```python
from build123d import *

# Parameters (mm, degrees)
EXTRUDE_1_DEPTH     = 5
EXTRUDE_5_DEPTH     = 30
EXTRUDE_6_DEPTH     = 30
CUT_EXTRUDE_1_DEPTH = 50
EXTRUDE_7_DEPTH     = 10
EXTRUDE_9_DEPTH     = 100
CUT_EXTRUDE_2_DEPTH = 653.725056973
SKETCH_15_W         = 153.587108834
SKETCH_15_H         = 200
EXTRUDE_11_DEPTH    = 5


with BuildPart() as part:
    # 草图1 → 凸台-拉伸1 (new body)
    with BuildSketch(Plane(origin=(0, 0, 0), x_dir=(1, 0, 0), z_dir=(0, 1, 0))):
        Polygon((-505, -50), (-505, 220), (-425, 300), (425, 300), (505, 220), (505, -10), (505, -220), (425, -300), (-425, -300), (-505, -220), align=None)
    extrude(amount=EXTRUDE_1_DEPTH)

    # 草图5 → 凸台-拉伸5 (add)
    with BuildSketch(Plane(origin=(0, 5, 0), x_dir=(1, 0, 0), z_dir=(0, 1, 0))):
        Polygon((90, 0), (90, -10), (110, -10), (110, 10), (90, 10), align=None)
    extrude(amount=EXTRUDE_5_DEPTH)

    # 草图6 → 凸台-拉伸6 (add)
    with BuildSketch(Plane(origin=(0, 35, 0), x_dir=(1, 0, 0), z_dir=(0, 1, 0))):
        Polygon((100, -25), (125, -25), (125, 25), (75, 25), (75, -25), align=None)
    extrude(amount=EXTRUDE_6_DEPTH)

    # 草图7 → 切除-拉伸1 (cut)
    with BuildSketch(Plane(origin=(125, 0, 0), x_dir=(0, 0, -1), z_dir=(1, 0, 0))):
        Polygon((0, 57.5), (-7.5, 57.5), (-7.5, 42.5), (7.5, 42.5), (7.5, 57.5), align=None)
    extrude(amount=-CUT_EXTRUDE_1_DEPTH, mode=Mode.SUBTRACT)

    # 草图8 → 凸台-拉伸7 (add)
    with BuildSketch(Plane(origin=(0, 5, 0), x_dir=(1, 0, 0), z_dir=(0, 1, 0))):
        with BuildLine():
            Line((505, 0), (505, 150))
            Line((505, 150), (424.355957742, 150))
            ThreePointArc((424.355957742, 150), (480, 0), (424.355957742, -150))
            Line((424.355957742, -150), (505, -150))
            Line((505, -150), (505, 0))
        make_face()
    extrude(amount=EXTRUDE_7_DEPTH)

    # 草图12 → 凸台-拉伸9 (add)
    with BuildSketch(Plane(origin=(0, 5, 0), x_dir=(1, 0, 0), z_dir=(0, 1, 0))):
        Polygon((30, -90), (100, -90), (180, -90), (180, -100), (100, -100), (30, -100), align=None)
        Polygon((100, 100), (30, 100), (30, 90), (100, 90), (180, 90), (180, 100), align=None)
    extrude(amount=EXTRUDE_9_DEPTH)

    # 草图13 → 切除-拉伸2 (cut, through all)
    with BuildSketch(Plane.XY.offset(100)):
        Polygon((180, 105), (180, 72), (30, 105), align=None)
    extrude(amount=-CUT_EXTRUDE_2_DEPTH, mode=Mode.SUBTRACT)

    # 草图15 → 凸台-拉伸11 (add)
    with BuildSketch(Plane(origin=(23.418542541, 106.447920641, 0), x_dir=(0.9766444667050901, -0.21486178267511977, 0), z_dir=(0.21486178267511977, 0.9766444667050901, 0))):
        with Locations((83.532401237, 0)):
            Rectangle(SKETCH_15_W, SKETCH_15_H)
    extrude(amount=EXTRUDE_11_DEPTH)


solid = part.part
```
The model under review builds one solid part; all positions refer to its coordinate system, in mm. A direction names the side the tool comes from. Round coordinates to 2 decimals unless told otherwise and drop trailing zeros. Loops run counter-clockwise (first coordinate to the right, second up) from the corner with the lowest first, then second, coordinate; pieces in that order, holes last. Notation, with made-up numbers: M 89.5,-3 L 99.5,-3 A34 ccw 99.5,32 Z; hole C 31,20.25 d4. An arc over 180 degrees is marked long. Put each result on its own line as item: value.
Q1. Machinability: for faces 1 (the flat face through (105.024, 93.614, -1.4)), 2 (the flat face through (100, 20, 10)), 3 (the flat face through (100, 65, 0)), 4 (the flat face through (89, 35, 0)), 5 (the flat face through (-464, 2, 261)), which of the approach directions +Z, -Z, +X, -X, +Y, -Y give a long, thin tool a straight path to every point of the face, cutting with its end or side? Answer none if there is none.
Result set:
face 1: +Z, -Z, +X, +Y
face 2: -X
face 3: +X, -X
face 4: none
face 5: +Z, -X, +Y, -Y
Q2. Consider section B-B, the plane z = 79. Give the boundary of the cut face in (x, y), then the cut area to 3 significant figures.
Result set:
outline: M -505,0 L 505,0 L 505,15 L 466.01,15 L 466.01,5 L -505,5 Z; M 30,105 L 180,72 L 181.07,76.88 L 31.07,109.88 Z
area: 6,210 mm²
Q3. Mouldability with a two-part tool opening along X and no side actions: class faces 6 (the flat face through (100, 20, -10)), 7 (the flat face through (110, 20, 0)), 8 (the flat face through (466, 2, 259)) as released by +X, released by -X, zero draft, split by the parting line, or undercut.
Result set:
face 6: zero draft
face 7: undercut
face 8: released by +X
Q4. Consider section D-D, the plane z = 204. Give the boundary of the cut face in (x, y), then the cut area to 3 significant figures.
Result set:
outline: M -505,0 L 505,0 L 505,5 L -505,5 Z
area: 5,050 mm²
Q5. Consider section C-C, the plane x = -274.5. Give the boundary of the cut face in (y, z), then the cut area to 3 significant figures.
Result set:
outline: M 0,-300 L 5,-300 L 5,300 L 0,300 Z
area: 3,000 mm²
Q6. For pin 1 (6 mm diameter, centred on y = 20.5, z = 2.5, fed in from +X); pin 2 (8 mm diameter, centred on y = 67, z = -96, fed in from -X); pin 3 (6 mm diameter, centred on x = 100, y = 14, fed in from +Z), all flat-tipped, find the tip position at first contact; note any pin that passes through.
Result set:
pin 1: stops at x = 110
pin 2: stops at x = 30
pin 3: stops at z = 100
Q7. To check wall thickness, follow L1, parallel to Z at x = 80, y = 24; L2, parallel to Y at x = 352, z = 249.5; L3, parallel to X at y = 63.5, z = -1.5. State the ranges of each line that lie inside material, in increasing order.
Result set:
L1: z = -100 to -90, 90 to 100
L2: y = 0 to 5
L3: x = 75 to 125
Q8. Consider section A-A, the plane y = 25. Give the boundary of the cut face in (x, z), then the cut area to 3 significant figures.
Result set:
outline: M 30,-100 L 180,-100 L 180,-90 L 30,-90 Z; M 30,90 L 180,90 L 180,100 L 30,100 Z; M 90,-10 L 110,-10 L 110,10 L 90,10 Z
area: 3,400 mm²
